Study the drawing (mm; zero at the part's minimum x, y, z) and answer. A direction names the side the tool comes from. Coordinates: 2 decimals unless noted, no trailing zeros. Order: outer loops, then holes, each group sorted by start corner. A loop starts at its lowest first (then second) coordinate and runs counter-clockwise, first axis right, second up. Notation, with made-up numbers: M 71.25,-27.5 L 76.25,-27.5 A27 cw 76.25,-11.5 Z; hole C 54.5,-29.75 d9. An arc over 180 degrees is marked long. Put each result on its own line as item: value.
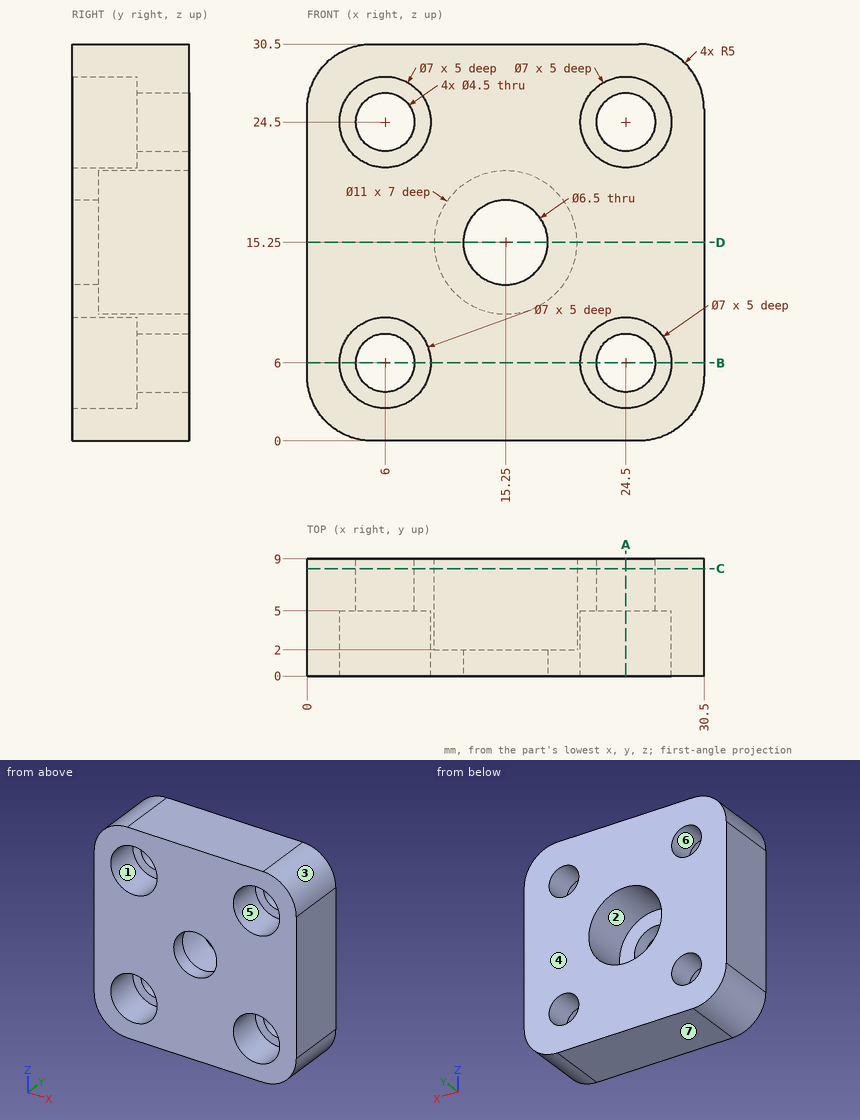
Q1. Find section A-A on x = 24.5. Write down the section's boundary in (y, z), plus the area to 4 significant figures.
Answers below:
outline: M 0,0 L 9,0 L 9,3.75 L 5,3.75 L 5,2.5 L 0,2.5 Z; M 0,9.5 L 5,9.5 L 5,8.25 L 9,8.25 L 9,22.25 L 5,22.25 L 5,21 L 0,21 Z; M 0,28 L 5,28 L 5,26.75 L 9,26.75 L 9,30.5 L 0,30.5 Z
area: 168.5 mm^2
Q2. A tool of negligible diameter and unlimited length cuts with its end or side. For the marked faces 1, 2 and 3, from which of +Z, -Z, +X, -X, +Y, -Y can it reach the whole face along a straight path? Write none if from no direction.
Answers below:
face 1: -Y
face 2: +Y
face 3: +Z, +X, +Y, -Y
Q3. For a pull along Z with two mould halves and no side action, classify the marked faces 4, 5, 6 and 7 as +Z half, -Z half, draft (parallel to the pull), parting line (faces both ways), or undercut.
Answers below:
face 4: draft
face 5: undercut
face 6: undercut
face 7: -Z half
Q4. Consider line 1 along Z through (x, y) = (24.5, 4.05); line 2 along X through (y, z) = (6.6, 24.5). Determine where each line is inside the solid, lowest interval first.
Answers below:
line 1: z = 0 to 2.5, 9.5 to 21, 28 to 30.5
line 2: x = 0 to 3.75, 8.25 to 22.25, 26.75 to 30.5
Q5. Find section B-B on z = 6. Write down the section's boundary in (x, y), plus the area to 4 significant figures.
Answers below:
outline: M 0,0 L 2.5,0 L 2.5,5 L 3.75,5 L 3.75,9 L 0,9 Z; M 8.25,5 L 9.5,5 L 9.5,0 L 21,0 L 21,5 L 22.25,5 L 22.25,9 L 8.25,9 Z; M 26.75,5 L 28,5 L 28,0 L 30.5,0 L 30.5,9 L 26.75,9 Z
area: 168.5 mm^2
Q6. Given pin 1 (6.5 mm diameter, centred on x = 24.5, z = 24.5, fed in from -Y); pin 2 (4 mm diameter, centred on x = 24.5, z = 6, fed in from -Y), each flat-ended and moving along its own axis, determine where each tip first touches the part or whether it passes through.
Answers below:
pin 1: stops at y = 5
pin 2: passes through
Q7. Find section D-D on z = 15.25. Write down the section's boundary in (x, y), plus the area to 4 significant figures.
Answers below:
outline: M 0,0 L 12,0 L 12,2 L 9.75,2 L 9.75,9 L 0,9 Z; M 18.5,0 L 30.5,0 L 30.5,9 L 20.75,9 L 20.75,2 L 18.5,2 Z
area: 184.5 mm^2
Q8. Find section C-C on y = 8.25. Write down the section's boundary in (x, z).
Answers below:
outline: M 0,5 A5 ccw 5,0 L 25.5,0 A5 ccw 30.5,5 L 30.5,25.5 A5 ccw 25.5,30.5 L 5,30.5 A5 ccw 0,25.5 Z; hole C 6,6 d4.5; hole C 6,24.5 d4.5; hole C 15.25,15.25 d11; hole C 24.5,6 d4.5; hole C 24.5,24.5 d4.5
